For this review, take the finished solid that the model builds, in its own axes (mm). Face numbers are marked on the shaded views. Give positions to 0.01 mm unless a question says otherwise; leave off trailing zeros. Write each loop counter-clockwise with the first axis right and the second up, starting at its lowest first coordinate (ties: lowest second). Pieces come first, ordered by that corner, then holes.
Q1. Mouldability with a two-part tool opening along Y and no side actions: class the marked faces 1 and 2 as released by +Y, released by -Y, zero draft, split by the parting line, or undercut.
Q2. We need section A-A (y = 67.5). Write out the cut boundary in (x, z), then the cut area to 3 significant figures.
Q3. We need section C-C (y = 22.5). Write out the cut boundary in (x, z).
Q4. We need section B-B (x = -100). Write out the cut boundary in (y, z), then the cut area to 3 significant figures.
Q5. For line 1 (Y direction, x = 100, z = 1.5); line 2 (X direction, y = -69.5, z = 1); line 3 (Y direction, x = -31, z = 2.5), list the stretches that pass through material, from the lowest coordinate up.
Q6. We need section D-D (x = 63). Write out the cut boundary in (y, z), then the cut area to 3 significant figures.
Q7. Insertion check: P1, Ø3.5, axis at x = 33.33, y = 67.5, coming from the +Z side; P2, Ø5, axis at x = -13, y = -9, coming from the +Z side. Each pin has a flat end and moves straight along its axis. Give the tip position at first contact, or say it passes through.
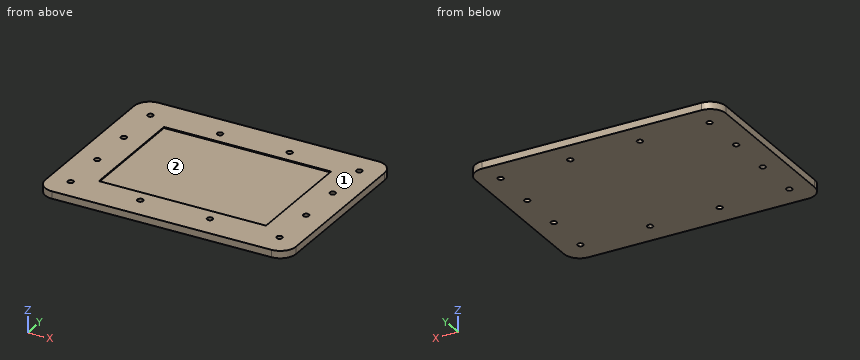
```python
from build123d import *

# Parameters (mm, degrees)
SKETCH003_W         = 240
SKETCH003_H         = 180
PAD002_DEPTH        = 7
SKETCH004_R         = 2.75
POCKET_DEPTH        = 7.001
LINEARPATTERN_COUNT = 4
LINEARPATTERN_PITCH = 66.666667
SKETCH041_R         = 2.75
POCKET001_DEPTH     = 607.164311
SKETCH_W            = 160
SKETCH_H            = 110
POCKET002_DEPTH     = 1
FILLET_R            = 15


with BuildPart() as part:
    # Sketch003 → Pad002 (new body)
    with BuildSketch(Plane.XY):
        Rectangle(SKETCH003_W, SKETCH003_H)
    extrude(amount=PAD002_DEPTH)

    # Sketch004 (on Face6 of Pad002) → Pocket (cut, through all)
    with BuildSketch(Plane.XY.offset(7)):
        with Locations((-100, 67.5)):
            Circle(SKETCH004_R)
        with Locations((-100, -67.5)):
            Circle(SKETCH004_R)
    pocket = extrude(amount=-POCKET_DEPTH, mode=Mode.SUBTRACT)

    # LinearPattern: Pocket ×4
    with Locations(*[(i * LINEARPATTERN_PITCH, 0, 0) for i in range(1, LINEARPATTERN_COUNT)]):
        add(pocket, mode=Mode.SUBTRACT)

    # Sketch041 (on Face5 of LinearPattern) → Pocket001 (cut, through all)
    with BuildSketch(Plane.XY.offset(7)):
        with Locations((-100, 22.5)):
            Circle(SKETCH041_R)
        with Locations((-100, -22.5)):
            Circle(SKETCH041_R)
    pocket001 = extrude(amount=-POCKET001_DEPTH, mode=Mode.SUBTRACT)

    # Mirrored: Pocket001 across YZ
    add(pocket001.mirror(Plane.YZ), mode=Mode.SUBTRACT)

    # Sketch (on Face5 of Mirrored) → Pocket002 (cut)
    with BuildSketch(Plane.XY.offset(7)):
        Rectangle(SKETCH_W, SKETCH_H)
    extrude(amount=-POCKET002_DEPTH, mode=Mode.SUBTRACT)

    # Fillet
    fillet_edges = [part.edges().sort_by_distance(p)[0] for p in [
        (-120, -90, 3.5),
        (-120, 90, 3.5),
        (120, 90, 3.5),
        (120, -90, 3.5),
    ]]
    fillet(fillet_edges, radius=FILLET_R)


solid = part.part
```
Computed:
1. face 1: zero draft
1. face 2: undercut
2. outline: (-120, 0) - (-102.75, 0) - (-102.75, 7) - (-120, 7) - close; (-97.25, 0) - (-36.08, 0) - (-36.08, 7) - (-97.25, 7) - close; (-30.58, 0) - (30.58, 0) - (30.58, 7) - (-30.58, 7) - close; (36.08, 0) - (97.25, 0) - (97.25, 7) - (36.08, 7) - close; (102.75, 0) - (120, 0) - (120, 7) - (102.75, 7) - close
2. area: 1,530 mm2
3. outline: (-120, 0) - (-102.75, 0) - (-102.75, 7) - (-120, 7) - close; (-97.25, 0) - (97.25, 0) - (97.25, 7) - (80, 7) - (80, 6) - (-80, 6) - (-80, 7) - (-97.25, 7) - close; (102.75, 0) - (120, 0) - (120, 7) - (102.75, 7) - close
4. outline: (-90, 0) - (-70.25, 0) - (-70.25, 7) - (-90, 7) - close; (-64.75, 0) - (-25.25, 0) - (-25.25, 7) - (-64.75, 7) - close; (-19.75, 0) - (19.75, 0) - (19.75, 7) - (-19.75, 7) - close; (25.25, 0) - (64.75, 0) - (64.75, 7) - (25.25, 7) - close; (70.25, 0) - (90, 0) - (90, 7) - (70.25, 7) - close
4. area: 1,110 mm2
5. line 1: y = -90 to -70.25, -64.75 to -25.25, -19.75 to 19.75, 25.25 to 64.75, 70.25 to 90
5. line 2: x = -120 to -101.89, -98.11 to -35.22, -31.45 to 31.45, 35.22 to 98.11, 101.89 to 120
5. line 3: y = -90 to -68.96, -66.04 to 66.04, 68.96 to 90
6. outline: (-90, 0) - (90, 0) - (90, 7) - (55, 7) - (55, 6) - (-55, 6) - (-55, 7) - (-90, 7) - close
6. area: 1,150 mm2
7. P1: passes through
7. P2: stops at z = 6
